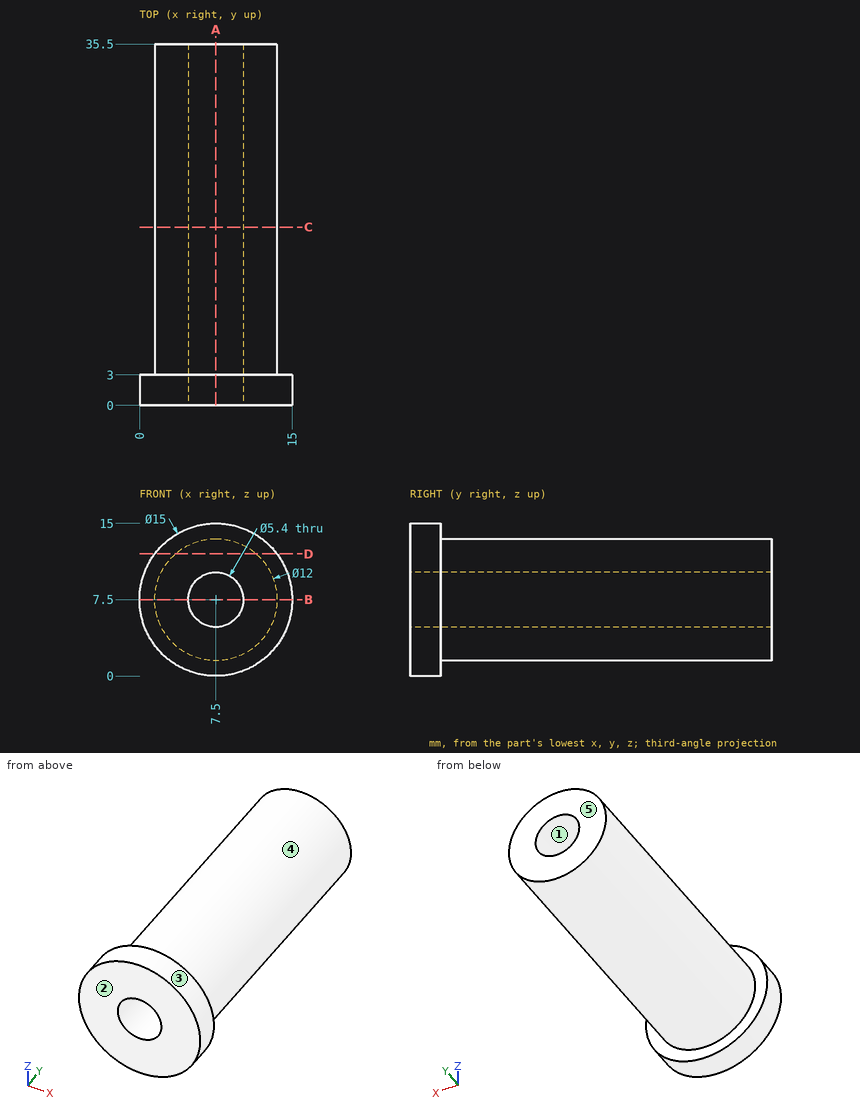
Input: dimensioned drawing with shaded views. Units: mm. Origin: part minimum x, y, z. A direction names the side the tool comes from. Coordinates: 2 decimals unless noted, no trailing zeros. Loops run counter-clockwise (first coordinate to the right, second up) from the corner with the lowest first, then second, coordinate; pieces in that order, holes last. Notation, with made-up numbers: (78, -14.5) -> (82, -14.5) arc R35 ccw to (82, 17.5) -> close; hole circle Ø9 at (82.5, -8.5). An arc over 180 degrees is marked (long way). Use a Markdown table: item, result. Add a question column.
(1) Section query A-A, the plane x = 7.5. Return loops of the section in (y, z), plus the area to 3 significant figures.
(2) Mould query, pull axis X, two halves, no side actions, for the marked faces 1, 2 and 3. Classes: pulls with the +X half, pulls with the -X half, needs draft (parallel to the pull), parting line crosses it, or undercut.
(3) Access query for the marked faces 4 and 5. Directions: +Z, -Z, +X, -X, +Y, -Y. A direction counts if a zero-diameter tool reaches every point of the face in a straight line with its end or side. Return the directions, or none.
(4) Section query C-C, the plane y = 17.5. Return loops of the section in (x, z).
(5) Section query D-D, the plane z = 12. Return loops of the section in (x, y), plus the area to 3 significant figures.
(6) Line query: line 1 along X through (y, z) = (17, 7.5); line 2 along Y through (x, z) = (12.75, 4); line 3 along Z through (x, y) = (5.5, 32.5). Output: solid intervals per line, ascending.
(7) Section query B-B, the plane z = 7.5. Return loops of the section in (x, y), plus the area to 3 significant figures.
(8) Pin query (flat end, axial travel): pin 1 Ø1 at (y, z) = (18.5, 7.5) entering from -X; pin 2 Ø4.5 at (x, z) = (7.5, 7.5) entering from -Y; pin 3 Ø3 at (x, y) = (6.5, 16) entering from +Z; pin 4 Ø6 at (x, y) = (12.5, 24.5) entering from -Z. Return the tip coordinate at first contact, or that it passes through.
Answer:
| question | item | result |
|---|---|---|
| 1 | outline | (0, 0) -> (3, 0) -> (3, 1.5) -> (35.5, 1.5) -> (35.5, 4.8) -> (0, 4.8) -> close; (0, 10.2) -> (35.5, 10.2) -> (35.5, 13.5) -> (3, 13.5) -> (3, 15) -> (0, 15) -> close |
| 1 | area | 243 mm^2 |
| 2 | face 1 | undercut |
| 2 | face 2 | needs draft |
| 2 | face 3 | parting line crosses it |
| 3 | face 4 | +Y |
| 3 | face 5 | +Z, -Z, +X, -X, +Y |
| 4 | outline | circle Ø12 at (7.5, 7.5); hole circle Ø5.4 at (7.5, 7.5) |
| 5 | outline | (1.5, 0) -> (13.5, 0) -> (13.5, 3) -> (11.47, 3) -> (11.47, 35.5) -> (3.53, 35.5) -> (3.53, 3) -> (1.5, 3) -> close |
| 5 | area | 294 mm^2 |
| 6 | line 1 | x = 1.5 to 4.8, 10.2 to 13.5 |
| 6 | line 2 | y = 0 to 3 |
| 6 | line 3 | z = 1.84 to 5.69, 9.31 to 13.16 |
| 7 | outline | (0, 0) -> (4.8, 0) -> (4.8, 35.5) -> (1.5, 35.5) -> (1.5, 3) -> (0, 3) -> close; (10.2, 0) -> (15, 0) -> (15, 3) -> (13.5, 3) -> (13.5, 35.5) -> (10.2, 35.5) -> close |
| 7 | area | 243 mm^2 |
| 8 | pin 1 | stops at x = 1.5 |
| 8 | pin 2 | passes through |
| 8 | pin 3 | stops at z = 13.5 |
| 8 | pin 4 | stops at z = 1.84 |
